Geometry: see drawing. Coordinates: mm, zero at the bounding-box minimum. Coordinates: 2 decimals unless noted, no trailing zeros. Loops run counter-clockwise (first coordinate to the right, second up) from the corner with the lowest first, then second, coordinate; pieces in that order, holes last. Notation, with made-up numbers: (85.5, -38.5) - (138.5, -38.5) arc R19 cw to (138.5, -6.5) - close; hole circle Ø10 at (15.5, 75.25). An arc over 180 degrees is marked (long way). Answer in a Markdown table with one row per item.
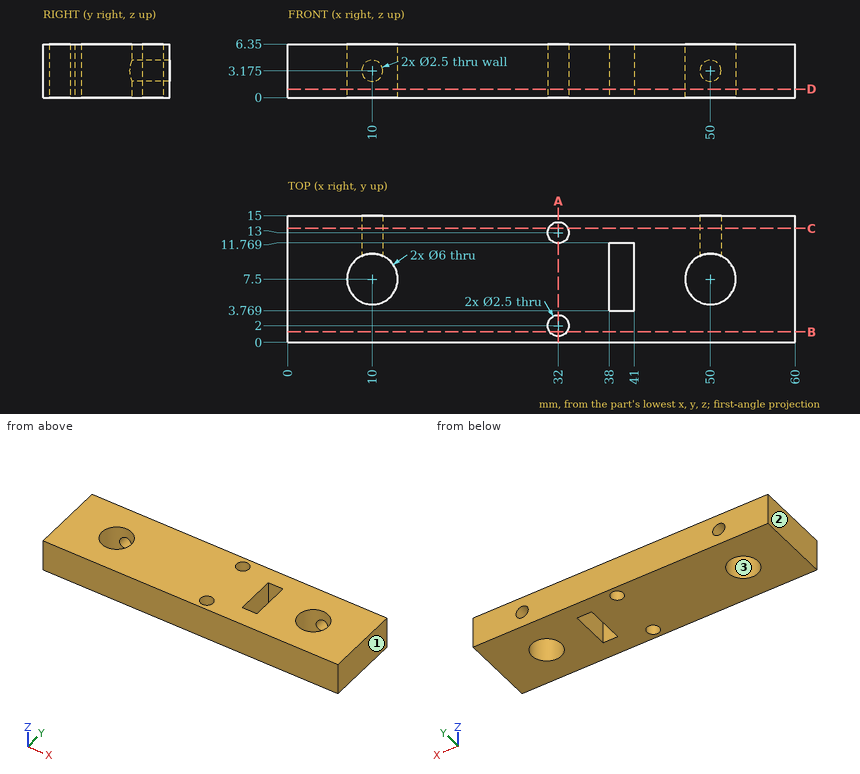
(1) Cut plane D-D on z = 1. Output: boundary loops of the cut face in (x, y).
Verdict:
| item | result |
|---|---|
| outline | (0, 0) - (60, 0) - (60, 15) - (0, 15) - close; hole circle Ø6 at (10, 7.5); hole circle Ø2.5 at (32, 2); hole circle Ø2.5 at (32, 13); hole (38, 3.77) - (41, 3.77) - (41, 11.77) - (38, 11.77) - close; hole circle Ø6 at (50, 7.5) |
(2) Cut plane A-A on x = 32. Output: boundary loops of the cut face in (y, z).
Verdict:
| item | result |
|---|---|
| outline | (0, 0) - (0.75, 0) - (0.75, 6.35) - (0, 6.35) - close; (3.25, 0) - (11.75, 0) - (11.75, 6.35) - (3.25, 6.35) - close; (14.25, 0) - (15, 0) - (15, 6.35) - (14.25, 6.35) - close |
(3) Ray query, probe 1 along Y at (x, z) = (32, 1.5); probe 2 along Y at (x, z) = (39, 1.5); probe 3 along X at (y, z) = (7.75, 4). Return the intervals inside material, ascending.
Verdict:
| item | result |
|---|---|
| probe 1 | y = 0 to 0.75, 3.25 to 11.75, 14.25 to 15 |
| probe 2 | y = 0 to 3.77, 11.77 to 15 |
| probe 3 | x = 0 to 7.01, 12.99 to 38, 41 to 47.01, 52.99 to 60 |
(4) Cut plane C-C on y = 13.5. State how many separate pieces and enclosed holes the cut face has, then the cut area to 3 significant figures.
Verdict:
| item | result |
|---|---|
| separate pieces | 2 |
| enclosed holes | 2 |
| area | 357 mm² |
(5) Cut plane B-B on y = 1.25. Output: boundary loops of the cut face in (x, z), then the cut area to 3 significant figures.
Verdict:
| item | result |
|---|---|
| outline | (0, 0) - (31, 0) - (31, 6.35) - (0, 6.35) - close; (33, 0) - (60, 0) - (60, 6.35) - (33, 6.35) - close |
| area | 368 mm² |
(6) Pull-direction query (X, two-part tool) for the marked faces 1, 2 and 3; classes: pulls with the +X half, pulls with the -X half, needs draft (parallel to the pull), parting line crosses it, or undercut.
Verdict:
| item | result |
|---|---|
| face 1 | pulls with the +X half |
| face 2 | pulls with the -X half |
| face 3 | undercut |
